The model under review builds one solid part; all positions refer to its coordinate system, in mm. Face numbers are marked on the shaded views. A direction names the side the tool comes from. Round coordinates to 2 decimals unless told otherwise and drop trailing zeros. Write each loop counter-clockwise with the first axis right and the second up, starting at its lowest first coordinate (ties: lowest second). Pieces come first, ordered by that corner, then holes. Notation, with made-up numbers: (81.25, 85.5) - (114.25, 85.5) arc R32 cw to (114.25, 120.5) - close; hole circle Ø1 at (1.25, 40.5). An arc over 180 degrees is marked (long way). Write each question's results on one line, items separated by ' | '.
```python
from build123d import *

# Parameters (mm, degrees)
F0_R     = 8.5
F1_DEPTH = 4
F2_R     = 5
F3_DEPTH = 100
F6_R     = 0.5
F7_DEPTH = 118.6


with BuildPart() as f1:
    # F0 (on Top) → F1 (new body)
    with BuildSketch(Plane.XY):
        Circle(F0_R)
    extrude(amount=F1_DEPTH)

    # F2 (on Top) → F3 (join)
    with BuildSketch(Plane.XY):
        Circle(F2_R)
    extrude(amount=F3_DEPTH)

    # F4 (on Right) → F5 (revolve)
    with BuildSketch(Plane.YZ):
        with BuildLine():
            Line((0, 104.582576), (0, 100))
            Line((0, 100), (5, 100))
            ThreePointArc((5, 100), (4.1833, 102.738613), (2, 104.582576))
            Line((2, 104.582576), (0, 104.582576))
        make_face()
        with BuildLine():
            ThreePointArc((0, 105), (1.021548, 104.894532), (2, 104.582576))
            Line((2, 104.582576), (1, 109.582576))
            Line((1, 109.582576), (0, 109.582576))
            Line((0, 109.582576), (0, 105))
        make_face()
        with BuildLine():
            Line((0, 105), (0, 104.582576))
            Line((0, 104.582576), (2, 104.582576))
            ThreePointArc((2, 104.582576), (1.021548, 104.894532), (0, 105))
        make_face()
    revolve(axis=Axis((0, 0, 104.791288), (0, 0, -1)))

    # F6 (on face) → F7 (cut)
    with BuildSketch(Plane(origin=(0, 0, 0), x_dir=(1, 0, 0), z_dir=(0, 0, -1))):
        Circle(F6_R)
    extrude(amount=-F7_DEPTH, mode=Mode.SUBTRACT)


solid = f1.part
```
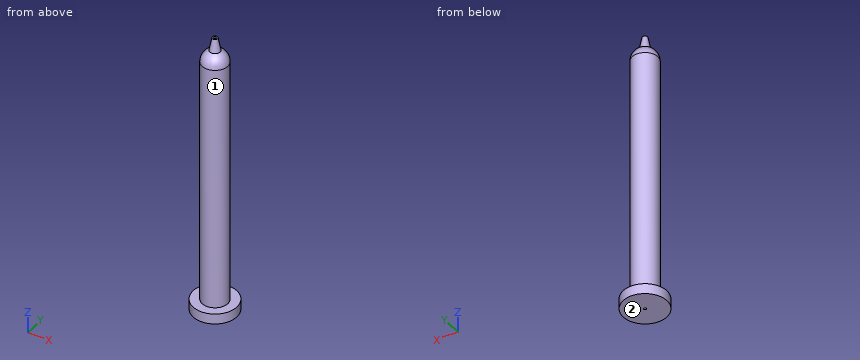
Q1. We need section C-C (y = 6.75). State the section outline as (x, z) points, plus the area to 3 significant figures.
Evaluation:
outline: (-5.17, 0) - (5.17, 0) - (5.17, 4) - (-5.17, 4) - close | area: 41.3 mm^2
Q2. We need section B-B (x = 6). State the section outline as (y, z) points.
Evaluation:
outline: (-6.02, 0) - (6.02, 0) - (6.02, 4) - (-6.02, 4) - close
Q3. For probe 1 along Y at (x, z) = (0, 25.5); probe 2 along Z at (x, y) = (-2.25, -5.25), list the stretches that pass through material, from the lowest coordinate up.
Evaluation:
probe 1: y = -5 to -0.5, 0.5 to 5 | probe 2: z = 0 to 4
Q4. Insertion check: P1, Ø1.5, axis at y = -6.5, z = 14.5, coming from the -X side; P2, Ø10, axis at x = -1.5, y = 1, coming from the -Z side; P3, Ø1, axis at x = -1, z = 41.5, coming from the +Y side; P4, Ø8, axis at y = 0.5, z = 98, coming from the +X side. Each pin has a flat end and moves straight along its axis. Give the tip position at first contact, or say it passes through.
Evaluation:
P1: passes through | P2: stops at z = 0 | P3: stops at y = 4.97 | P4: stops at x = 5
Q5. Tool access review of the marked faces 1 and 2: name each direction out of +Z, -Z, +X, -X, +Y, -Y from which nothing blocks a thin tool from reaching the whole face with its end or side.
Evaluation:
face 1: +Z | face 2: -Z, +X, -X, +Y, -Y
Q6. We need section A-A (z = 9). State the section outline as (x, y) points, plus the area to 3 significant figures.
Evaluation:
outline: circle Ø10 at (0, 0); hole circle Ø1 at (0, 0) | area: 77.8 mm^2
